For this review, take the finished solid that the model builds, in its own axes (mm). A direction names the side the tool comes from. Coordinates: 2 decimals unless noted, no trailing zeros. Loops run counter-clockwise (first coordinate to the right, second up) from the corner with the lowest first, then second, coordinate; pieces in that order, holes last. Notation, with made-up numbers: (-5.75, 43.25) -> (24.25, 43.25) arc R16 cw to (24.25, 63.25) -> close; hole circle Ø7 at (56.25, 38). An arc over 180 degrees is marked (long way). One line per item, written item: value.
from build123d import *

# Parameters (mm, degrees)
EXTRUDE_1_DEPTH      = 21
EXTRUDE_1_DEPTH_BACK = 21
CUT_EXTRUDE_1_REACH  = 90.549
SKETCH_3_R           = 2.5
EXTRUDE_2_DEPTH      = 19


with BuildPart() as part:
    # Sketch 1 → Extrude 1 (new, two sides: drawn at the far end of the back side and taken through both)
    with BuildSketch(Plane.XY.offset(-EXTRUDE_1_DEPTH_BACK)):
        Polygon((0, 53), (0, 0), (70, 0), (70, 3), (3, 3), (3, 53), align=None)
    extrude(amount=EXTRUDE_1_DEPTH + EXTRUDE_1_DEPTH_BACK)

    # Sketch 2 → Cut-Extrude 1 (cut, up to next)
    with BuildSketch(Plane(origin=(0, 3, 0), x_dir=(1, 0, 0), z_dir=(0, 1, 0)), mode=Mode.PRIVATE) as cut_extrude_1_sk1:
        with BuildLine():
            Line((12, -11), (60, -11))
            ThreePointArc((60, -11), (64, -15), (60, -19))
            Line((60, -19), (12, -19))
            ThreePointArc((12, -19), (8, -15), (12, -11))
        make_face()
    cut_extrude_1_tool1 = extrude(cut_extrude_1_sk1.sketch, amount=-CUT_EXTRUDE_1_REACH, mode=Mode.PRIVATE) & part.part
    # Sketch 2 → Cut-Extrude 1 (cut, up to next)
    with BuildSketch(Plane(origin=(0, 3, 0), x_dir=(1, 0, 0), z_dir=(0, 1, 0)), mode=Mode.PRIVATE) as cut_extrude_1_sk2:
        with BuildLine():
            Line((12, 11), (60, 11))
            ThreePointArc((60, 11), (64, 15), (60, 19))
            Line((60, 19), (12, 19))
            ThreePointArc((12, 19), (8, 15), (12, 11))
        make_face()
    cut_extrude_1_tool2 = extrude(cut_extrude_1_sk2.sketch, amount=-CUT_EXTRUDE_1_REACH, mode=Mode.PRIVATE) & part.part
    add(cut_extrude_1_tool1.solids().sort_by_distance((36, 3, 15))[0], mode=Mode.SUBTRACT)
    add(cut_extrude_1_tool2.solids().sort_by_distance((36, 3, -15))[0], mode=Mode.SUBTRACT)

    # Sketch 3 → Extrude 2 (add)
    with BuildSketch(Plane.ZY):
        with Locations(Location((0, 28, 0), (0, 0, 270))):
            Circle(SKETCH_3_R)
    extrude(amount=EXTRUDE_2_DEPTH)


solid = part.part
1. Take a section at D-D, the plane z = 4. Give the boundary of the cut face in (x, y).
Return value:
outline: (0, 0) -> (70, 0) -> (70, 3) -> (3, 3) -> (3, 53) -> (0, 53) -> close
2. Insertion check: pin 1 Ø12 at (y, z) = (7, 1.5) entering from -X; pin 2 Ø4 at (y, z) = (10.5, 9.5) entering from +X; pin 3 Ø2 at (x, z) = (21, -8) entering from +Y. Each pin has a flat end and moves straight along its axis. Give the tip position at first contact, or say it passes through.
Return value:
pin 1: stops at x = 0
pin 2: stops at x = 3
pin 3: stops at y = 3
3. To check wall thickness, follow probe 1 along Y at (x, z) = (23.5, 4.5). State the ranges of the line that lie inside material, in increasing order. Write a range as from..to.
Return value:
probe 1: y = 0..3
4. Take a section at C-C, the plane y = 28. Give the boundary of the cut face in (x, z).
Return value:
outline: (-19, -2.5) -> (0, -2.5) -> (0, -21) -> (3, -21) -> (3, 21) -> (0, 21) -> (0, 2.5) -> (-19, 2.5) -> close
5. The part is to be moulded in two halves that separate along Z. For faces 1 (the cylindrical face through (-9.4, 30.5, 0.1)), 2 (the flat face through (2, 53, 0)), 3 (the flat face through (36, 2, 11)), 4 (the flat face through (19, 1, -21)), say which applies: pulls with the +Z half, pulls with the -Z half, needs draft (parallel to the pull), parting line crosses it, or undercut.
Return value:
face 1: parting line crosses it
face 2: needs draft
face 3: undercut
face 4: pulls with the -Z half
6. Take a section at A-A, the plane x = 40. Give the boundary of the cut face in (y, z).
Return value:
outline: (0, -21) -> (3, -21) -> (3, -19) -> (0, -19) -> close; (0, -11) -> (3, -11) -> (3, 11) -> (0, 11) -> close; (0, 19) -> (3, 19) -> (3, 21) -> (0, 21) -> close
7. Take a section at B-B, the plane z = -15. Give the boundary of the cut face in (x, y), and give its area (3 significant figures).
Return value:
outline: (0, 0) -> (8, 0) -> (8, 3) -> (3, 3) -> (3, 53) -> (0, 53) -> close; (64, 0) -> (70, 0) -> (70, 3) -> (64, 3) -> close
area: 192 mm2
8. For faces 5 (the cylindrical face through (8, 2, 15)), 6 (the flat face through (3, 28, 0)), 7 (the flat face through (19, 1, 21)), list the 3-axis set-ups (+Z, -Z, +X, -X, +Y, -Y) from which the entire face can be reached by the end or side of a thin tool; tool diameter is ignored.
Return value:
face 5: +Y, -Y
face 6: +Z, -Z, +X, +Y
face 7: +Z, +X, -X, +Y, -Y
